Design review of the part shown in the three views and the two pictorial views. Dimensions are in mm from the part's minimum x, y and z. A direction names the side the tool comes from. Give positions to 0.01 mm unless a question says otherwise; leave off trailing zeros. Loops run counter-clockwise (first coordinate to the right, second up) from the corner with the lowest first, then second, coordinate; pieces in that order, holes last. Notation, with made-up numbers: (-32, 88) - (-9, 88) arc R20 ccw to (-9, 93) - close; hole circle Ø7 at (-27.5, 0). An arc over 180 degrees is marked (long way). Answer as a JSON object with one key per item and string values.
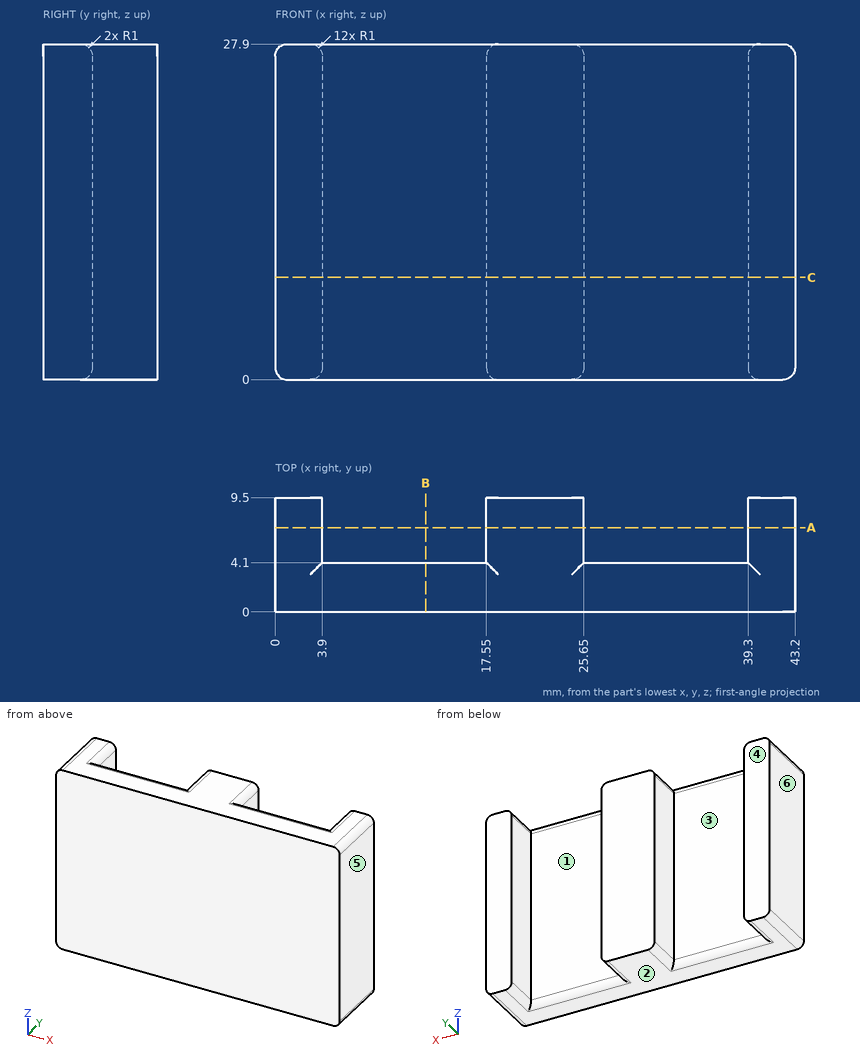
Q1. To check wall thickness, follow probe 1 along X at (y, z) = (5, 5.5); probe 2 along Y at (x, z) = (34, 19); probe 3 along Z at (x, y) = (39.5, 4). State the ranges of each line that lie inside material, in increasing order. Write a range as [from, to].
Results:
{"probe 1": "x = [0, 3.9], [17.55, 25.65], [39.3, 43.2]", "probe 2": "y = [0, 4.1]", "probe 3": "z = [0.4, 27.5]"}
Q2. Consider section C-C, the plane z = 8.5. State the section outline as (x, y) points, plus the area to 3 significant figures.
Results:
{"outline": "(0, 0) - (43.2, 0) - (43.2, 9.5) - (39.3, 9.5) - (39.3, 4.1) - (25.65, 4.1) - (25.65, 9.5) - (17.55, 9.5) - (17.55, 4.1) - (3.9, 4.1) - (3.9, 9.5) - (0, 9.5) - close", "area": "263 mm^2"}
Q3. Consider section B-B, the plane x = 12.5. State the section outline as (y, z) points, plus the area to 3 significant figures.
Results:
{"outline": "(0, 0) - (3.1, 0) arc R1 ccw to (4.1, 1) - (4.1, 26.9) arc R1 ccw to (3.1, 27.9) - (0, 27.9) - close", "area": "114 mm^2"}
Q4. The part is to be moulded in two halves that separate along X. For the marked faces 3, 4, 5 and 6, say which applies: +X half, -X half, draft (parallel to the pull), parting line (faces both ways), or undercut.
Results:
{"face 3": "undercut", "face 4": "draft", "face 5": "+X half", "face 6": "-X half"}
Q5. Clearance check with a flat-ended pin moving along its axis: pin 1 Ø1.5 at (x, z) = (11, 7) entering from +Y. State where the tip first meets the part, or that it passes through.
Results:
{"pin 1": "stops at y = 4.1"}
Q6. For the marked faces 1 and 2, list the 3-axis set-ups (+Z, -Z, +X, -X, +Y, -Y) from which the entire face can be reached by the end or side of a thin tool; tool diameter is ignored.
Results:
{"face 1": "+Z, -Z, +Y", "face 2": "-Z, +X, -X, +Y, -Y"}
Q7. Consider section A-A, the plane y = 7. State the section outline as (x, z) points.
Results:
{"outline": "(0, 1) arc R1 ccw to (1, 0) - (2.9, 0) arc R1 ccw to (3.9, 1) - (3.9, 26.9) arc R1 ccw to (2.9, 27.9) - (1, 27.9) arc R1 ccw to (0, 26.9) - close; (17.55, 1) arc R1 ccw to (18.55, 0) - (24.65, 0) arc R1 ccw to (25.65, 1) - (25.65, 26.9) arc R1 ccw to (24.65, 27.9) - (18.55, 27.9) arc R1 ccw to (17.55, 26.9) - close; (39.3, 1) arc R1 ccw to (40.3, 0) - (42.2, 0) arc R1 ccw to (43.2, 1) - (43.2, 26.9) arc R1 ccw to (42.2, 27.9) - (40.3, 27.9) arc R1 ccw to (39.3, 26.9) - close"}
